Answer from the drawing. Dimensions are ordinates in mm from the lowest x, y and z of the part. A direction names the side the tool comes from. Coordinates: 2 decimals unless noted, no trailing zeros. Order: outer loops, then holes, each group sorted by start corner. A loop starts at its lowest first (then second) coordinate and runs counter-clockwise, first axis right, second up. Notation, with made-up numbers: (-28, 69) -> (7, 69) arc R31 ccw to (7, 101) -> close; hole circle Ø2 at (60.25, 62.25). An arc over 180 degrees is marked (long way). Answer in a Markdown table with one row per item.
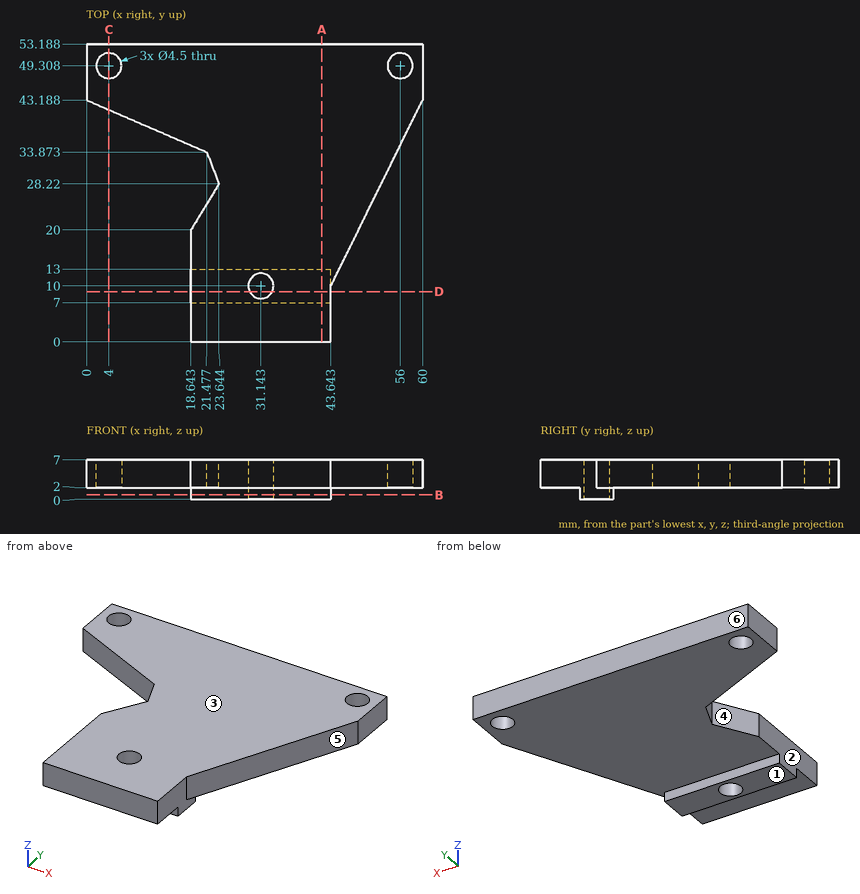
Q1. Given pin 1 (6 mm diameter, centred on x = 20, y = 33.5, fed in from -Z); pin 2 (1 mm diameter, centred on x = 32, z = 1, fed in from -Y); pin 3 (2 mm diameter, centred on x = 36, z = 0.5, fed in from +Y); pin 4 (2.5 mm diameter, centred on x = 4, y = 49.31, fed in from +Z), each flat-ended and moving along its own axis, determine where each tip first touches the part or whether it passes through.
Outcome:
| item | result |
|---|---|
| pin 1 | z = 2 |
| pin 2 | y = 7 |
| pin 3 | y = 13 |
| pin 4 | through |
Q2. The part is cut by section B-B (z = 0.75). Write down the section's boundary in (x, y).
Outcome:
| item | result |
|---|---|
| outline | (18.64, 7) -> (43.64, 7) -> (43.64, 13) -> (18.64, 13) -> close; hole circle Ø4.5 at (31.14, 10) |
Q3. The part is cut by section C-C (x = 4). Write down the section's boundary in (y, z).
Outcome:
| item | result |
|---|---|
| outline | (41.45, 2) -> (47.06, 2) -> (47.06, 7) -> (41.45, 7) -> close; (51.56, 2) -> (53.19, 2) -> (53.19, 7) -> (51.56, 7) -> close |
Q4. The part is cut by section D-D (y = 9). Write down the section's boundary in (x, z).
Outcome:
| item | result |
|---|---|
| outline | (18.64, 0) -> (29.13, 0) -> (29.13, 7) -> (18.64, 7) -> close; (33.16, 0) -> (43.64, 0) -> (43.64, 7) -> (33.16, 7) -> close |
Q5. Consider line 1 (X direction, y = 49, z = 2.75); line 2 (Z direction, x = 14.5, y = 45); line 3 (X direction, y = 6, z = 5.25). Determine where each line is inside the solid, lowest interval first.
Outcome:
| item | result |
|---|---|
| line 1 | 0 to 1.77, 6.23 to 53.77, 58.23 to 60 |
| line 2 | 2 to 7 |
| line 3 | 18.64 to 43.64 |
Q6. For the marked faces 1 and 2, determine the directions among +Z, -Z, +X, -X, +Y, -Y from which every point of the face is accessible in a straight line to the end or side of a thin tool.
Outcome:
| item | result |
|---|---|
| face 1 | -Z, +X, -X, +Y, -Y |
| face 2 | +Z, -Z, -X, -Y |
Q7. For a pull along Y with two mould halves and no side action, classify the marked faces 3, 4, 5 and 6 as pulls with the +Y half, pulls with the -Y half, needs draft (parallel to the pull), parting line crosses it, or undercut.
Outcome:
| item | result |
|---|---|
| face 3 | needs draft |
| face 4 | undercut |
| face 5 | pulls with the -Y half |
| face 6 | pulls with the +Y half |
Q8. The part is cut by section A-A (x = 42). Write down the section's boundary in (y, z).
Outcome:
| item | result |
|---|---|
| outline | (0, 2) -> (7, 2) -> (7, 0) -> (13, 0) -> (13, 2) -> (53.19, 2) -> (53.19, 7) -> (0, 7) -> close |
